Could you check a few things on this model? Use its own coordinates, in mm. Round coordinates to 2 decimals unless told otherwise and drop trailing zeros. Write each loop counter-clockwise with the first axis right and the second up, starting at its lowest first coordinate (ties: lowest second). Pieces come first, ordered by that corner, then holes. Notation, with made-up numbers: (-20.5, -25) -> (23.5, -25) arc R23 ccw to (23.5, 4) -> close; hole circle Ø10 at (66.25, 17). An arc over 180 degrees is marked (long way). Answer in a Markdown table with one row per item. Add a question column.
```python
from build123d import *

# Parameters (mm, degrees)
F0_R     = 19.05
F1_DEPTH = 901.7
F2_W     = 38.1
F2_H     = 57.15
F3_DEPTH = 25.4
F5_W     = 38.1
F5_H     = 57.15
F6_DEPTH = 25.4
F7_R     = 28.575
F7_R_2   = 19.05
F8_DEPTH = 31.75


with BuildPart() as f1:
    # F0 (on Right) → F1 (new body, symmetric)
    with BuildSketch(Plane.YZ):
        Circle(F0_R)
    extrude(amount=F1_DEPTH, both=True)

    # F2 (on Right) → F3 (join, symmetric)
    with BuildSketch(Plane.YZ):
        with Locations((0, 9.525)):
            Rectangle(F2_W, F2_H)
    extrude(amount=F3_DEPTH, both=True)

    # F5 (on offset) → F6 (join, symmetric)
    with BuildSketch(Plane.YZ.offset(630.2375)):
        with Locations((0, 9.525)):
            Rectangle(F5_W, F5_H)
    extrude(amount=F6_DEPTH, both=True)



with BuildPart() as f8:
    # F7 (on face) → F8 (new body)
    with BuildSketch(Plane.YZ.offset(901.7)):
        Circle(F7_R)
        Circle(F7_R_2, mode=Mode.SUBTRACT)
    extrude(amount=-F8_DEPTH)


with BuildPart() as f1_1:
    add(f1.part)

    add(f8.part)  # F9 merges F8
    # F9: F1, F8 across plane
    add(f1.part.mirror(Plane.YZ))
    add(f8.part.mirror(Plane.YZ))


solid = f1_1.part
```
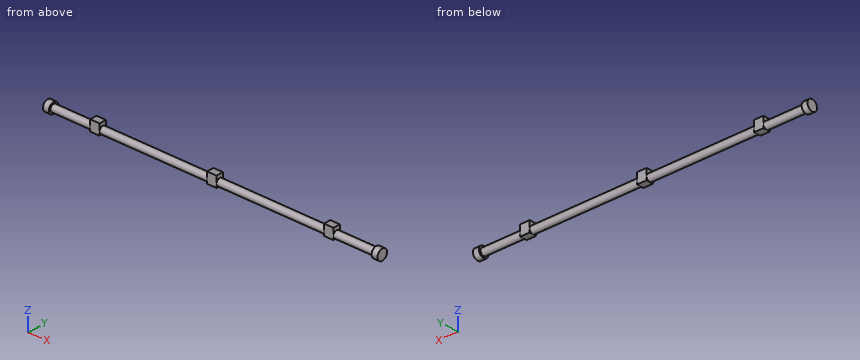
(1) Suppose I cut it at A-A, the plane x = -488.5. Please give me the cut outline in (y, z).
(2) For P1, Ø10, axis at x = 250.5, y = 8, coming from the -Z side; P2, Ø5, axis at x = -573, y = 6, coming from the +Z side; P3, Ø1.5, axis at x = 534.5, z = -15, coming from the +Y side, each with a flat end and sliding along its axis, tell me the tip position at first contact or that it passes through.
(3) I need wall thicknesses on L1, parallel to X at y = 3, z = 21.5; L2, parallel to X at y = -7, z = -24; L3, parallel to Y at x = -21.5, z = 33. Which ranges of each line are inside material? Lowest first, please.
Response:
| question | item | result |
|---|---|---|
| 1 | outline | circle Ø38.1 at (0, 0) |
| 2 | P1 | z = -18.81 |
| 2 | P2 | z = 18.73 |
| 2 | P3 | y = 12.64 |
| 3 | L1 | -901.7 to -869.95, -655.64 to -604.84, -25.4 to 25.4, 604.84 to 655.64, 869.95 to 901.7 |
| 3 | L2 | -901.7 to -869.95, 869.95 to 901.7 |
| 3 | L3 | -19.05 to 19.05 |
